Autodesk Inventor part; units mm, degrees
ref_plane "YZ Plane" through (0, 0, 0) normal (1, 0, 0) x (0, 1, 0)
ref_plane "XZ Plane" through (0, 0, 0) normal (0, 1, 0) x (-1, 0, 0)
ref_plane "XY Plane" through (0, 0, 0) normal (0, 0, 1) x (1, 0, 0)
sketch "Sketch5" plane through (0, 0, 0) normal (0, 1, 0) x (-1, 0, 0)
  line L0 (-22.225, 22.225) -> (-22.225, -22.225)
  line L1 (-22.225, -22.225) -> (22.225, -22.225)
  line L2 (22.225, -22.225) -> (22.225, 22.225)
  line L3 (22.225, 22.225) -> (-22.225, 22.225)
  line L4 (-22.225, 22.225) -> (22.225, -22.225) construction
  line L5 (-22.225, -22.225) -> (22.225, 22.225) construction
  point P0 (0, 0)
  dimension "d23" = 44.45
extrude "Extrusion3" add sketch "Sketch5" along normal blind 12.7
sketch "Sketch6" plane through (-22.225, 0, 22.225) normal (0, 0, 1) x (1, 0, 0)
  point P0 (22.225, 0)
  point P1 (22.225, 0)
hole "Hole2" at (0, 0, 22.225) direction (0, 0, -1) diameter 9.525 end through all
sketch "Sketch7" plane through (0, 12.7, 0) normal (0, 1, 0) x (1, 0, 0)
  line L0 (-22.225, 22.225) -> (-22.225, -22.225)
  line L1 (22.225, -22.225) -> (22.225, 22.225)
  line L2 (-22.225, -22.225) -> (22.225, -22.225)
  point P0 (0, 0)
  point P1 (-13.4938, 0)
  point P2 (13.4938, 0)
  dimension "d33" = 8.7312
  dimension "d34" = 8.7312
  dimension "d53" = 22.225
  dimension "d54" = 22.225
hole "Hole3" at (-13.4938, 12.7, 0) at (13.4938, 12.7, 0) direction (0, -1, 0) diameter 13.335 depth 6.096
sketch "Sketch8" plane through (0, 12.7, 0) normal (0, 1, 0) x (1, 0, 0)
  line L0 (-22.225, 22.225) -> (-22.225, -22.225)
  line L1 (22.225, -22.225) -> (22.225, 22.225)
  line L2 (-22.225, -22.225) -> (22.225, -22.225)
  point P0 (0, 0)
  point P1 (-13.4938, 0)
  point P2 (13.4938, 0)
  dimension "d42" = 8.7312
  dimension "d43" = 8.7312
  dimension "d51" = 22.225
  dimension "d52" = 22.225
hole "Hole4" at (-13.4938, 12.7, 0) at (13.4938, 12.7, 0) direction (0, -1, 0) diameter 5.1054 end through all
sketch "Sketch9" plane through (0, 0, 0) normal (0, -1, 0) x (1, 0, 0)
  line L0 (-13.4938, -13.4938) -> (13.4937, -13.4938) construction
  line L1 (13.4937, -13.4938) -> (13.4937, 13.4938) construction
  line L2 (13.4937, 13.4938) -> (-13.4938, 13.4938) construction
  line L3 (-13.4938, 13.4938) -> (-13.4938, -13.4938) construction
  line L4 (-13.4938, -13.4938) -> (13.4937, 13.4938) construction
  line L5 (13.4937, -13.4938) -> (-13.4938, 13.4938) construction
  line L6 (-4.7625, -22.225) -> (-22.225, -22.225) construction
  line L7 (-22.225, -22.225) -> (-22.225, 22.225) construction
  circle A0 centre (-13.4938, -13.4938) radius 2.54
  circle A1 centre (13.4937, -13.4938) radius 2.54
  circle A2 centre (13.4937, 13.4938) radius 2.54
  circle A3 centre (-13.4938, 13.4938) radius 2.54
  point P0 (0, 0)
  dimension "d55" = 8.7312
  dimension "d56" = 8.7312
  dimension "d57" = 5.08
extrude "Extrusion4" add sketch "Sketch9" along normal blind 10.16
fillet "Fillet1" radius 1.5875 4 edges at (-16.0338, -10.16, 13.4938) (10.9537, -10.16, 13.4938) (10.9537, -10.16, -13.4938) (-16.0338, -10.16, -13.4938)
equation "\"d23\" = basewidth"
equation "\"d24\" = heightOfTopSection"
equation "\"d26\" = topHoleDiam"
equation "\"d35\" = washerDiam"
equation "\"d40\" = depthForSocketHead"
equation "\"d55\" = edgeToBoltHole"
equation "\"d56\" = edgeToBoltHole"
equation "\"d57\" = supportHoleDiam"
equation "\"d58\" = supportHoleLength"
equation "\"bottomHoleDiam\" = 9.525"
equation "\"basewidth\" = 44.45"
equation "\"deltaBottomToTop\" = 25.4"
equation "\"d0\" = basewidth"
equation "\"d1\" = heightOfBottomHole"
equation "\"d2\" = 0"
equation "\"d3\" = bottomHoleDiam"
equation "\"d5\" = 0"
equation "\"topHoleDiam\" = 9.525"
equation "\"height\" = deltaBottomToTop + heightOfBottomHole + heightOfTopHole"
equation "\"heightOfTopSection\" = 12.7"
equation "\"edgeToBoltHole\" = -0.25 * bottomHoleDiam + 0.25 * basewidth"
equation "\"washerDiam\" = 13.335"
equation "\"depthForSocketHead\" = 6.096"
equation "\"heightOfTopSupport\" = 12.7"
equation "\"baseLength\" = 44.45"
equation "\"supportHoleDiam\" = 5.08"
equation "\"supportHoleLength\" = 10.16"
properties part number "TopOfSquareSupport" material "PC/ABS Plastic"
Work out the finished part from the listing and answer in its coordinate system (mm). A direction names the side the tool comes from. Coordinates: 2 decimals unless noted, no trailing zeros. Write each loop counter-clockwise with the first axis right and the second up, starting at its lowest first coordinate (ties: lowest second). Pieces come first, ordered by that corner, then holes.
Q1. Each of these flat-tipped pins is pushed along its axis until it touches: pin 1 Ø1 at (x, z) = (-14.5, 3) entering from +Y; pin 2 Ø8 at (x, z) = (-13.49, 0) entering from -Y. Where does it stop, or does it pass through?
Q2. Which of the six approach directions +Z, -Z, +X, -X, +Y, -Y give full straight-line access (tool end or side, diameter ignored) to faces 1 (the face through (11.478, -4.226, -11.948)), 2 (the face through (-20.1, 9.6, -0.9)), 3 (the face through (-14, -10.16, -13))?
Q3. A cutting plane is placed at B-B, the plane y = 1. Give the vertices of the cut face in (x, z) (3 decimals).
Q4. A cutting plane is placed at D-D, the plane y = 9. Give the vertices of the cut face in (x, z) (1 decimal).
Q5. A cutting plane is placed at A-A, the plane z = 0. Give the vertices of the cut face in (x, y) (1 decimal), then the cut area to 3 significant figures.
Q6. Determine the mould class of faces 4 (the face through (13, -10.16, 14)), 5 (the face through (-11.07, -4.23, 12.73)), 6 (the face through (-22.225, 6, 0)) for opening direction X: released by +X, released by -X, zero draft, split by the parting line, or undercut.
Q7. Find the intervals of material crossed by line 1 (Y direction, x = 16, z = -20); line 2 (Y direction, x = 16, z = -1); line 3 (Z direction, x = 12.5, y = 2) (3 decimals), in increasing order.
Q8. A cutting plane is placed at C-C, the plane x = 0. Give the vertices of the cut face in (y, z) (1 decimal), then the cut area to 3 significant figures.
Findings below:
1. pin 1: stops at y = 6.6
1. pin 2: stops at y = 0
2. face 1: -Y
2. face 2: +Y
2. face 3: +Z, -Z, +X, -X, -Y
3. outline: (-22.225, -22.225) - (-4.656, -22.225) - (-4.656, 22.225) - (-22.225, 22.225) - close; (4.656, -22.225) - (22.225, -22.225) - (22.225, 22.225) - (4.656, 22.225) - close; hole circle Ø5.105 at (-13.494, 0); hole circle Ø5.105 at (13.494, 0)
4. outline: (-22.2, -22.2) - (22.2, -22.2) - (22.2, 22.2) - (-22.2, 22.2) - close; hole circle Ø13.3 at (-13.5, 0); hole circle Ø13.3 at (13.5, 0)
5. outline: (-22.2, 0) - (-16, 0) - (-16, 6.6) - (-20.2, 6.6) - (-20.2, 12.7) - (-22.2, 12.7) - close; (-10.9, 0) - (-4.8, 0) arc R4.8 cw to (4.8, 0) - (10.9, 0) - (10.9, 6.6) - (6.8, 6.6) - (6.8, 12.7) - (-6.8, 12.7) - (-6.8, 6.6) - (-10.9, 6.6) - close; (16, 0) - (22.2, 0) - (22.2, 12.7) - (20.2, 12.7) - (20.2, 6.6) - (16, 6.6) - close
5. area: 299 mm2
6. face 4: zero draft
6. face 5: undercut
6. face 6: released by -X
7. line 1: y = 0 to 12.7
7. line 2: y = 0 to 6.6
7. line 3: z = -22.225 to -2.351, 2.351 to 22.225
8. outline: (4.8, -22.2) - (12.7, -22.2) - (12.7, 22.2) - (4.8, 22.2) - close
8. area: 353 mm2
